For this review, take the finished solid that the model builds, in its own axes (mm). A direction names the side the tool comes from. Coordinates: 2 decimals unless noted, no trailing zeros. Loops run counter-clockwise (first coordinate to the right, second up) from the corner with the lowest first, then second, coordinate; pieces in that order, holes last. Notation, with made-up numbers: M 62,-34 L 98,-34 A18 cw 98,-5 Z; hole C 48.25,49 d3. An arc over 180 degrees is marked long. Answer as a JSON object with one key per item and string values. Group by question number.
Item 1: Wall thickness on L1, parallel to X at y = 0, z = -14; L2, parallel to Y at x = 0, z = -18.5; L3, parallel to Y at x = 13, z = -13: over which ranges is each line inside the solid? List them lowest first. Write a range as from..to.
Item 2: Tool access review of faces 1 (the face through (-13.5, 22.4, 45)), 2 (the face through (-10.748, -26.79, 0.229)), 3 (the face through (-0.5, -28, -28)): name each direction out of +Z, -Z, +X, -X, +Y, -Y from which nothing blocks a thin tool from reaching the whole face with its end or side.
Item 3: Add section B-B (x = -12.5). State the section outline as (y, z) points.
Item 4: Add section C-C (z = 39.5). State the section outline as (x, y) points, then the cut area to 3 significant figures.
Item 5: Mouldability with a two-part tool opening along X and no side actions: class faces 4 (the face through (10.748, -26.79, -0.229)), 5 (the face through (-13.5, 22.4, -45)) as +X half, -X half, draft (parallel to the pull), parting line (faces both ways), or undercut.
Item 6: Insertion check: pin 1 (2 mm diameter, centred on y = 0.5, z = 28, fed in from -X); pin 2 (4.5 mm diameter, centred on y = -28.5, z = -30, fed in from -X); pin 3 (5 mm diameter, centred on x = 0.5, z = -25.5, fed in from +Y); pin 4 (3 mm diameter, centred on y = -27.5, z = -32, fed in from +X). Each pin has a flat end and moves straight along its axis. Give the tip position at first contact, or say it passes through.
Item 7: Add section A-A (y = 9). State the section outline as (x, z) points.
Item 8: Add section D-D (x = 7). State the section outline as (y, z) points.
from build123d import *

# Parameters (mm, degrees)
SKETCH009_R       = 30
SKETCH009_R_2     = 26
PAD002_DEPTH      = 45
PAD002_DEPTH_BACK = 45
SKETCH010_R       = 10.75
POCKET007_DEPTH   = 30.001
SKETCH027_W       = 1
SKETCH027_H       = 90
POCKET012_DEPTH   = 30.001


with BuildPart() as part:
    # Sketch009 → Pad002 (new body, two sides)
    with BuildSketch(Plane.XY) as pad002_sk:
        Circle(SKETCH009_R)
        Circle(SKETCH009_R_2, mode=Mode.SUBTRACT)
    extrude(amount=PAD002_DEPTH)
    extrude(pad002_sk.sketch, amount=-PAD002_DEPTH_BACK)

    # Sketch010 → Pocket007 (cut, through all)
    with BuildSketch(Plane.XZ):
        Circle(SKETCH010_R)
    extrude(amount=POCKET007_DEPTH, mode=Mode.SUBTRACT)

    # Sketch027 → Pocket012 (cut, through all)
    with BuildSketch(Plane.XZ):
        Rectangle(SKETCH027_W, SKETCH027_H)
    extrude(amount=POCKET012_DEPTH, mode=Mode.SUBTRACT)


solid = part.part
From the geometry:
{
 "1": {"L1": "x = -30..-26, 26..30", "L2": "y = 26..30", "L3": "y = -27.04..-22.52, 22.52..27.04"},
 "2": {"face 1": "+Z, +X, -X, +Y, -Y", "face 2": "-Y", "face 3": "+Z, -Z, -Y"},
 "3": {"outline": "M -27.27,-45 L -22.8,-45 L -22.8,45 L -27.27,45 Z; M 22.8,-45 L 27.27,-45 L 27.27,45 L 22.8,45 Z"},
 "4": {"outline": "M -0.5,-30 L -0.5,-26 A26 cw long 0.5,-26 L 0.5,-30 A30 ccw long Z", "area": "700 mm²"},
 "5": {"face 4": "undercut", "face 5": "draft"},
 "6": {"pin 1": "stops at x = -30", "pin 2": "stops at x = -14.52", "pin 3": "stops at y = 30", "pin 4": "stops at x = 14.97"},
 "7": {"outline": "M -28.62,-45 L -24.39,-45 L -24.39,45 L -28.62,45 Z; M 24.39,-45 L 28.62,-45 L 28.62,45 L 24.39,45 Z"},
 "8": {"outline": "M -29.17,-45 L -25.04,-45 L -25.04,-8.16 L -29.17,-8.16 Z; M -29.17,8.16 L -25.04,8.16 L -25.04,45 L -29.17,45 Z; M 25.04,-45 L 29.17,-45 L 29.17,45 L 25.04,45 Z"}
}
